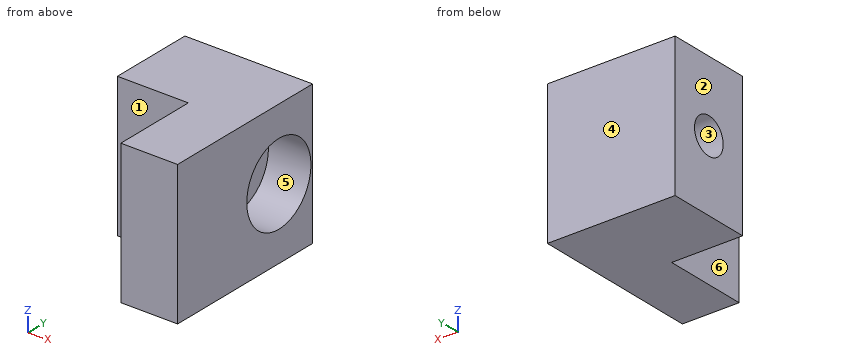
from build123d import *

# Parameters (mm, degrees)
BOSS_EXTRUDE1_DEPTH = 10


with BuildPart() as part:
    # Sketch1 → Boss-Extrude1 (new body)
    with BuildSketch(Plane.XY):
        Polygon((0, 0), (9, 0), (9, -12), (5, -12), (5, -6), (0, -6), align=None)
    extrude(amount=BOSS_EXTRUDE1_DEPTH)

    # Sketch4 → Cut-Revolve2 (revolve, cut)
    with BuildSketch(Plane(origin=(0, -3, 0), x_dir=(1, 0, 0), z_dir=(0, 1, 0)), mode=Mode.PRIVATE) as cut_revolve2_sk:
        Polygon((0, -5), (9, -5), (9, -2.15), (6, -2.15), (6, -3.725), (0, -3.725), align=None)
    revolve(cut_revolve2_sk.sketch.rotate(Axis((0, -3, 5), (1, 0, 0)), 270), axis=Axis((0, -3, 5), (1, 0, 0)), mode=Mode.SUBTRACT)


solid = part.part
Geometry: final body of the model. Coordinates: model frame, mm. Face numbers are marked on the shaded views. A direction names the side the tool comes from. Give positions to 0.01 mm unless a question says otherwise; leave off trailing zeros. Order: outer loops, then holes, each group sorted by start corner. A loop starts at its lowest first (then second) coordinate and runs counter-clockwise, first axis right, second up. Notation, with made-up numbers: (38.25, -39.5) -> (94.25, -39.5) arc R28 ccw to (94.25, -17.5) -> close; hole circle Ø3 at (3, -9). An arc over 180 degrees is marked (long way). Answer as a JSON object with one key per item and string values.
Q1. Material intervals for probe 1 along Z at (x, y) = (8.1, -3); probe 2 along Z at (x, y) = (3.5, -3) (3 decimals); probe 3 along Y at (x, z) = (8.4, 5), sorted ascending.
Entries:
{"probe 1": "z = 0 to 2.15, 7.85 to 10", "probe 2": "z = 0 to 3.725, 6.275 to 10", "probe 3": "y = -12 to -5.85, -0.15 to 0"}
Q2. Draft query along Y for the marked faces 3, 4, 5 and 6. Return one class per face: released by +Y, released by -Y, zero draft, split by the parting line, or undercut.
Entries:
{"face 3": "undercut", "face 4": "released by +Y", "face 5": "undercut", "face 6": "zero draft"}
Q3. Section C-C (x = 4.75). Output: boundary loops of the cut face in (y, z) (3 decimals).
Entries:
{"outline": "(-6, 0) -> (0, 0) -> (0, 10) -> (-6, 10) -> close; hole circle Ø2.55 at (-3, 5)"}
Q4. Section A-A (z = 5). Output: boundary loops of the cut face in (x, y) (3 decimals).
Entries:
{"outline": "(0, -6) -> (5, -6) -> (5, -12) -> (9, -12) -> (9, -5.85) -> (6, -5.85) -> (6, -4.275) -> (0, -4.275) -> close; (0, -1.725) -> (6, -1.725) -> (6, -0.15) -> (9, -0.15) -> (9, 0) -> (0, 0) -> close"}
Q5. Access query for the marked faces 1 and 2. Directions: +Z, -Z, +X, -X, +Y, -Y. A direction counts if a zero-diameter tool reaches every point of the face in a straight line with its end or side. Return the directions, or none.
Entries:
{"face 1": "+Z, -Z, -X, -Y", "face 2": "+Z, -Z, -X, +Y, -Y"}
Q6. Section D-D (z = 6.5). Output: boundary loops of the cut face in (x, y), plus the area to 3 significant figures.
Entries:
{"outline": "(0, -6) -> (5, -6) -> (5, -12) -> (9, -12) -> (9, -5.42) -> (6, -5.42) -> (6, -0.58) -> (9, -0.58) -> (9, 0) -> (0, 0) -> close", "area": "63.5 mm^2"}
Q7. Section B-B (y = -3). Output: boundary loops of the cut face in (x, z) (3 decimals).
Entries:
{"outline": "(0, 0) -> (9, 0) -> (9, 2.15) -> (6, 2.15) -> (6, 3.725) -> (0, 3.725) -> close; (0, 6.275) -> (6, 6.275) -> (6, 7.85) -> (9, 7.85) -> (9, 10) -> (0, 10) -> close"}
Q8. First-contact query: pin 1 (1.5 mm diameter, centred on x = 1.5, z = 6.5, fed in from -Y); pin 2 (1 mm diameter, centred on y = -4, z = 3.5, fed in from +X); pin 3 (5 mm diameter, centred on x = 1.5, y = -10.5, fed in from -Z); pin 4 (3 mm diameter, centred on y = -9.5, z = 9, fed in from -X). Flat tips, straight axial feed; report the tip coordinate or a pass-through.
Entries:
{"pin 1": "stops at y = -6", "pin 2": "stops at x = 6", "pin 3": "passes through", "pin 4": "stops at x = 5"}
